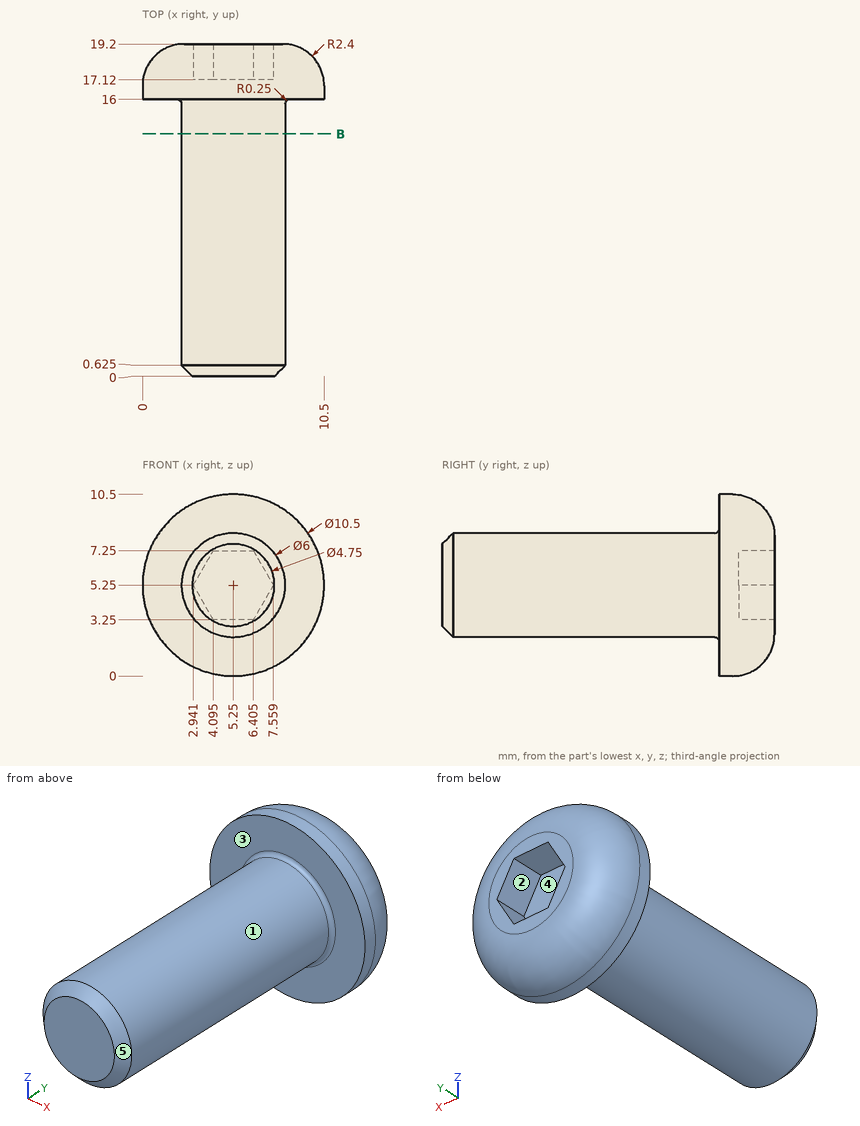
Source: three-view drawing plus pictorial views. Frame: mm from the lowest corner of the part. A direction names the side the tool comes from. Round coordinates to 2 decimals unless told otherwise and drop trailing zeros. Loops run counter-clockwise (first coordinate to the right, second up) from the corner with the lowest first, then second, coordinate; pieces in that order, holes last.
Q1. Section B-B on y = 14. Return loops of the section in (x, z), plus the area to 3 significant figures.
Q2. Pin query (flat end, axial travel): P1, Ø3, axis at x = 3.5, y = 6.5, coming from the -Z side; P2, Ø1, axis at x = 5, y = 18, coming from the -Z side; P3, Ø2, axis at x = 5, z = 5, coming from the +Y side. Return the tip coordinate at first contact, or that it passes through.
Q3. Access query for the marked faces 4 and 5. Directions: +Z, -Z, +X, -X, +Y, -Y. A direction counts if a zero-diameter tool reaches every point of the face in a straight line with its end or side. Return the directions, or none.
Q4. Material intervals for L1, parallel to Y at x = 5.75, z = 6.75; L2, parallel to Z at x = 5.25, y = 10.25; L3, parallel to X at y = 5.5, z = 3 (1 decimal), sorted ascending.
Q5. Pull-direction query (Z, two-part tool) for the marked faces 1, 2 and 3; classes: released by +Z, released by -Z, zero draft, split by the parting line, or undercut.
Evaluation:
1. outline: circle Ø6 at (5.25, 5.25)
1. area: 28.3 mm2
2. P1: stops at z = 2.26
2. P2: stops at z = 0.11
2. P3: stops at y = 17.12
3. face 4: +Y
3. face 5: -Y
4. L1: y = 0 to 17.12
4. L2: z = 2.25 to 8.25
4. L3: x = 3.3 to 7.2
5. face 1: split by the parting line
5. face 2: undercut
5. face 3: zero draft
